from build123d import *

# Parameters (mm, degrees)
IZIM1_R                     = 27
Y_KSEKLIK_EKSTR_ZYON1_DEPTH = 15
PAH1_SIZE                   = 10
PAH1_SIZE2                  = 17.320508076
RADYUS1_R                   = 10
RADYUS2_R                   = 4
RADYUS3_R                   = 4
IZIM2_R                     = 10
KES_EKSTR_ZYON1_DEPTH       = 2


with BuildPart() as part:
    # Çizim1 → Yükseklik-Ekstrüzyon1 (new body)
    with BuildSketch(Plane(origin=(0, 0, 0), x_dir=(1, 0, 0), z_dir=(0, 1, 0))):
        with Locations(Location((0, 0, 0), (0, 0, 270))):
            Circle(IZIM1_R)
    extrude(amount=Y_KSEKLIK_EKSTR_ZYON1_DEPTH)

    # Pah1
    pah1_edges = [part.edges().sort_by_distance(p)[0] for p in [
        (0, 15, -27),
    ]]
    pah1_side = [part.faces().sort_by_distance(p)[0] for p in [
        (0, 7.5, -27),
    ]]
    chamfer(pah1_edges, length=PAH1_SIZE, length2=PAH1_SIZE2, reference=pah1_side[0])

    # Radyus1
    radyus1_edges = [part.edges().sort_by_distance(p)[0] for p in [
        (0, 15, -9.679491924),
    ]]
    fillet(radyus1_edges, radius=RADYUS1_R)

    # Radyus2
    radyus2_edges = [part.edges().sort_by_distance(p)[0] for p in [
        (0, 5, -27),
    ]]
    fillet(radyus2_edges, radius=RADYUS2_R)

    # Radyus3
    # the kernel refuses this fillet: 4 mm, written as the material it takes off along each edge
    with BuildSketch(Plane(origin=(0, 0, 0), x_dir=(0, 0, 1), z_dir=(-1, 0, 0))) as radyus3_piece_1:
        with BuildLine():
            CenterArc((23.220386989, 4), RADYUS3_R, 270, 70.891973705)
            Line((23.220386989, 0), (23.220386989, -0.08))
            Line((23.220386989, -0.08), (27, -0.08))
            Line((27, -0.08), (27.08, 0))
            ThreePointArc((27.08, 0), (27.08, 1.345299462), (27.075591492, 2.664410902))
            Line((27.075591492, 2.664410902), (26.999999247, 2.690598923))
        make_face()
    revolve(axis=Axis((0, 0, 0), (0, 1, 0)), mode=Mode.SUBTRACT)

    # Çizim2 → Kes-Ekstrüzyon1 (cut)
    with BuildSketch(Plane.XZ):
        with Locations(Location((0, 0, 0), (0, 0, 270))):
            Circle(IZIM2_R)
    extrude(amount=-KES_EKSTR_ZYON1_DEPTH, mode=Mode.SUBTRACT)


solid = part.part
Could you check a few things on this model? Use its own coordinates, in mm. A direction names the side the tool comes from. Coordinates: 2 decimals unless noted, no trailing zeros. Write each loop counter-clockwise with the first axis right and the second up, starting at its lowest first coordinate (ties: lowest second). Pieces come first, ordered by that corner, then holes. Notation, with made-up numbers: (42, -20.5) - (99, -20.5) arc R20 ccw to (99, 2.5) - close; hole circle Ø4 at (5.25, -8). An arc over 180 degrees is marked (long way). Write item = value, one per line.
1) Suppose I cut it at A-A on y = 9.25. Please give me the cut outline in (x, z).
Result set:
outline = circle Ø39.28 at (0, 0)
2) For faces 1 (the flat face through (-5, 0, 10)), 2 (the flat face through (0, 2, 0)), which set-ups out of +Z, -Z, +X, -X, +Y, -Y let a thin tool reach every point of the face, with its end or its side?
Result set:
face_1 = +Z, -Z, +X, -X, -Y
face_2 = -Y
3) Will these pins go through, and if not, where does the flat tip stop? pin 1 Ø2 at (x, y) = (6, 5) entering from -Z; pin 2 Ø1.5 at (y, z) = (9, -2.5) entering from -X; pin 3 Ø8 at (y, z) = (8.5, -8) entering from -X.
Result set:
pin_1 = -26.16
pin_2 = -21.23
pin_3 = -25.59
4) We'd pull the mould along Z, two halves only. Please class faces 3 (the conical face through (3.794, 13.296, 12.048)), 4 (the cylindrical face through (-9.76, 0.99, 2.17)), 5 (the flat face through (0, 15, 0)): +Z half, -Z half, draft (parallel to the pull), parting line (faces both ways), or undercut.
Result set:
face_3 = parting line
face_4 = undercut
face_5 = draft
5) Please list where these lines run through material, in increasing order: line 1 (X direction, y = 1.1, z = 0); line 2 (X direction, y = 1.5, z = 0); line 3 (Y direction, x = 16, z = 9.5). Write a range as [from, to].
Result set:
line_1 = [-25.98, -10], [10, 25.98]
line_2 = [-26.34, -10], [10, 26.34]
line_3 = [0, 9.85]
